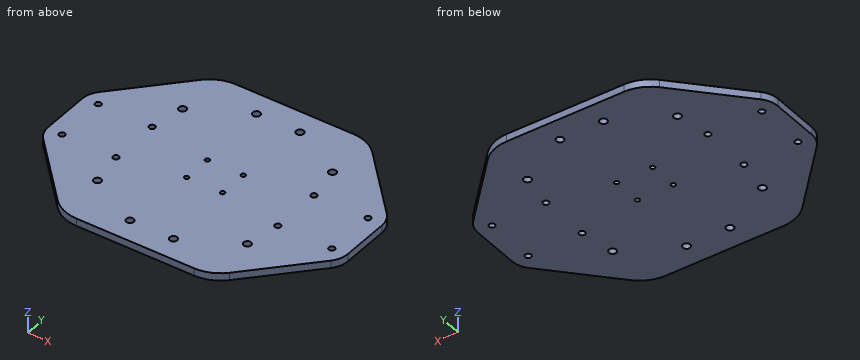
```python
from build123d import *

# Parameters (mm, degrees)
CROQUIS1_W              = 200
CROQUIS1_H              = 150.1
CROQUIS1_R              = 2.5
SALIENTE_EXTRUIR1_DEPTH = 5
CROQUIS2_R              = 1.5
CROQUIS2_R_2            = 2
CORTAR_EXTRUIR1_DEPTH   = 10
CORTAR_EXTRUIR2_DEPTH   = 400


with BuildPart() as part:
    # Croquis1 → Saliente-Extruir1 (new body)
    with BuildSketch(Plane.XY):
        with Locations((100, 5.648844896)):
            Rectangle(CROQUIS1_W, CROQUIS1_H)
        with Locations((85.5, 65.198844896)):
            Circle(CROQUIS1_R, mode=Mode.SUBTRACT)
        with Locations((114.5, 65.198844896)):
            Circle(CROQUIS1_R, mode=Mode.SUBTRACT)
        with Locations((50, 45.698844896)):
            Circle(CROQUIS1_R, mode=Mode.SUBTRACT)
        with Locations((150, 45.698844896)):
            Circle(CROQUIS1_R, mode=Mode.SUBTRACT)
        with Locations((150, -34.401155104)):
            Circle(CROQUIS1_R, mode=Mode.SUBTRACT)
        with Locations((114.5, -53.901155104)):
            Circle(CROQUIS1_R, mode=Mode.SUBTRACT)
        with Locations((85.5, -53.901155104)):
            Circle(CROQUIS1_R, mode=Mode.SUBTRACT)
        with Locations((50, -34.401155104)):
            Circle(CROQUIS1_R, mode=Mode.SUBTRACT)
    extrude(amount=SALIENTE_EXTRUIR1_DEPTH)

    # Croquis2 → Cortar-Extruir1 (cut)
    with BuildSketch(Plane.XY.offset(5)):
        with Locations((88, 15.398844896)):
            Circle(CROQUIS2_R)
        with Locations((112, 15.398844896)):
            Circle(CROQUIS2_R)
        with Locations((88, -4.101155104)):
            Circle(CROQUIS2_R)
        with Locations((112, -4.101155104)):
            Circle(CROQUIS2_R)
        with Locations((10, 22.648844896)):
            Circle(CROQUIS2_R_2)
        with Locations((46, 22.648844896)):
            Circle(CROQUIS2_R_2)
        with Locations((46, -11.351155104)):
            Circle(CROQUIS2_R_2)
        with Locations((10, -11.351155104)):
            Circle(CROQUIS2_R_2)
        with Locations((190, -11.351155104)):
            Circle(CROQUIS2_R_2)
        with Locations((154, -11.351155104)):
            Circle(CROQUIS2_R_2)
        with Locations((154, 22.648844896)):
            Circle(CROQUIS2_R_2)
        with Locations((190, 22.648844896)):
            Circle(CROQUIS2_R_2)
    extrude(amount=-CORTAR_EXTRUIR1_DEPTH, mode=Mode.SUBTRACT)

    # Croquis3 → Cortar-Extruir2 (cut)
    with BuildSketch(Plane(origin=(0, 0, 0), x_dir=(-1, 0, 0), z_dir=(0, 0, -1))):
        with BuildLine():
            Line((-195.915748263, 31.98223599), (-157.401555296, 72.845794728))
            ThreePointArc((-157.401555296, 72.845794728), (-149.116372199, 78.651772224), (-139.208641525, 80.698844896))
            Line((-139.208641525, 80.698844896), (-200, 80.698844896))
            Line((-200, 80.698844896), (-200, 21.694066091))
            ThreePointArc((-200, 21.694066091), (-198.941596464, 27.2286743), (-195.915748263, 31.98223599))
        make_face()
        with BuildLine():
            Line((0, 80.698844896), (-60.791358475, 80.698844896))
            ThreePointArc((-60.791358475, 80.698844896), (-50.883627801, 78.651772224), (-42.598444704, 72.845794728))
            Line((-42.598444704, 72.845794728), (-4.084251737, 31.98223599))
            ThreePointArc((-4.084251737, 31.98223599), (-1.058403536, 27.2286743), (0, 21.694066091))
            Line((0, 21.694066091), (0, 80.698844896))
        make_face()
        with BuildLine():
            Line((0, -69.401155104), (0, -10.396376298))
            ThreePointArc((0, -10.396376298), (-1.058403536, -15.930984508), (-4.084251737, -20.684546197))
            Line((-4.084251737, -20.684546197), (-42.598444704, -61.548104935))
            ThreePointArc((-42.598444704, -61.548104935), (-50.883627801, -67.354082431), (-60.791358475, -69.401155104))
            Line((-60.791358475, -69.401155104), (0, -69.401155104))
        make_face()
        with BuildLine():
            ThreePointArc((-195.915748263, -20.684546197), (-198.941596464, -15.930984508), (-200, -10.396376298))
            Line((-200, -10.396376298), (-200, -69.401155104))
            Line((-200, -69.401155104), (-139.208641525, -69.401155104))
            ThreePointArc((-139.208641525, -69.401155104), (-149.116372199, -67.354082431), (-157.401555296, -61.548104935))
            Line((-157.401555296, -61.548104935), (-195.915748263, -20.684546197))
        make_face()
    extrude(amount=-CORTAR_EXTRUIR2_DEPTH, mode=Mode.SUBTRACT)


solid = part.part
```
Source: CAD feature listing. Evaluate the final solid. Frame: model axes, mm. Coordinates: 2 decimals unless noted, no trailing zeros. Loops run counter-clockwise (first coordinate to the right, second up) from the corner with the lowest first, then second, coordinate; pieces in that order, holes last. Notation, with made-up numbers: M 21.25,37 L 69.25,37 A27 ccw 69.25,67 Z; hole C -27.5,-0.5 d1. An arc over 180 degrees is marked long. Use CSV: the item, a comma, the result in double quotes.
(1) Cut plane C-C on y = -28. Return loops of the section in (x, z), and give its area (3 significant figures).
Answers follow:
outline,"M 10.98,0 L 189.02,0 L 189.02,5 L 10.98,5 Z"
area,"890 mm²"
(2) Cut plane A-A on z = 3.1. Give the number of separate pieces and of enclosed holes in the cut face, and give its area (3 significant figures).
Answers follow:
separate pieces,"1"
enclosed holes,"20"
area,"24,400 mm²"
(3) Cut plane B-B on x = 166.5. Return loops of the section in (y, z).
Answers follow:
outline,"M -51.89,0 L 63.19,0 L 63.19,5 L -51.89,5 Z"
(4) Line query: line 1 (Y direction, x = 85.5, z = 1.85); line 2 (X direction, y = 24, z = 2.1); line 3 (X direction, y = 16.5, z = 0.7). Output: solid intervals per line, ascending. Write a range as [from, to].
Answers follow:
line 1,"[-69.4, -56.4], [-51.4, 62.7], [67.7, 80.7]"
line 2,"[0.18, 8.53], [11.47, 44.53], [47.47, 152.53], [155.47, 188.53], [191.47, 199.82]"
line 3,"[0, 86.98], [89.02, 110.98], [113.02, 200]"
(5) Contact query for flat-ended pins moving along their axis: pin 1 (1 mm diameter, centred on y = -33, z = 1.5, fed in from -X); pin 2 (1.5 mm diameter, centred on x = 158.5, z = 1.5, fed in from -Y); pin 3 (2.5 mm diameter, centred on x = 190, y = 22.65, fed in from -Z); pin 4 (2 mm diameter, centred on x = 156.5, z = 4, fed in from +Y). Output: stop coordinate, or through.
Answers follow:
pin 1,"x = 15.22"
pin 2,"y = -61.18"
pin 3,"through"
pin 4,"y = 74.66"
